Input: part model. Units: mm. Frame: model coordinates. A direction names the side the tool comes from. Coordinates: 2 decimals unless noted, no trailing zeros. One line per question, with ' | ' between items.
from build123d import *

# Parameters (mm, degrees)
F1_DEPTH  = 3.175
F2_W      = 25.4
F2_H      = 6.35
F3_DEPTH  = 12.7
F5_DEPTH  = 6.35
F7_DEPTH  = 6.35
F10_DEPTH = 6.35
F13_R     = 0.873125
F14_DEPTH = 25.4


with BuildPart() as f1:
    # F0 (on Front) → F1 (new body, symmetric)
    with BuildSketch(Plane.XZ):
        Polygon((3.175, 15.875), (0, 15.875), (-3.175, 15.875), (-12.7, 0), (12.7, 0), align=None)
        Polygon((12.7, -6.35), (12.7, 0), (-12.7, 0), (-12.7, -6.35), (0, -6.35), align=None)
        Polygon((0, -15.875), (12.7, -6.35), (0, -6.35), align=None)
        Polygon((0, -6.35), (-12.7, -6.35), (0, -15.875), align=None)
    extrude(amount=F1_DEPTH, both=True)

    # F2 (on face) → F3 (join)
    with BuildSketch(Plane.XZ.offset(3.175)):
        with Locations((0, -3.175)):
            Rectangle(F2_W, F2_H)
    extrude(amount=F3_DEPTH)

    # F4 (on face) → F5 (join)
    with BuildSketch(Plane(origin=(7.62, 0, -10.16), x_dir=(0.8, 0, 0.6), z_dir=(0.6, 0, -0.8))):
        Polygon((-9.525, 3.175), (6.35, 3.175), (6.35, 15.875), align=None)
    extrude(amount=-F5_DEPTH)

    # F6 (on face) → F7 (join)
    with BuildSketch(Plane(origin=(-7.62, 0, -10.16), x_dir=(0.8, 0, -0.6), z_dir=(-0.6, 0, -0.8))):
        Polygon((-6.35, 15.875), (-6.35, 3.175), (9.525, 3.175), align=None)
    extrude(amount=-F7_DEPTH)

    # F9 (on 3pt) → F10 (join)
    with BuildSketch(Plane(origin=(0, -8.763, -11.684), x_dir=(1, 0, 0), z_dir=(0, -0.6, -0.8))):
        Polygon((0, -6.9850953296), (12.700131163, 8.8898520917), (-12.699984014, 8.8898520917), align=None)
    extrude(amount=-F10_DEPTH)

    # F13 (on 3pt) → F14 (cut)
    with BuildSketch(Plane(origin=(0, -9.525, 9.525), x_dir=(1, 0, 0), z_dir=(0, -0.7071067812, 0.7071067812))):
        with Locations((0, 3.3772722036)):
            Circle(F13_R)
    extrude(amount=-F14_DEPTH, mode=Mode.SUBTRACT)


solid = f1.part
Item 1: Contact query for flat-ended pins moving along their axis: P1, Ø6, axis at y = -3.5, z = -12.5, coming from the +X side; P2, Ø12.5, axis at x = 0, z = 10.5, coming from the -Y side (3 decimals); P3, Ø1.1, axis at x = 0.5, y = -3.5, coming from the -Z side. Output: stop coordinate, or through.
Data:
P1: x = 8.5 | P2: y = -3.175 | P3: z = -15.85
Item 2: Access query for faces 1 (the face through (0, -3.175, 6)), 2 (the face through (0, -4, -6.35)), 3 (the face through (12.7, -6, -3)). Directions: +Z, -Z, +X, -X, +Y, -Y. A direction counts if a zero-diameter tool reaches every point of the face in a straight line with its end or side. Return the directions, or none.
Data:
face 1: +Z, +X, -X, -Y | face 2: none | face 3: +Z, -Z, +X, +Y, -Y
Item 3: Draft query along X for faces 4 (the face through (0, -9, 0)), 5 (the face through (8, -0.04, 7.83)), 6 (the face through (-7.9, 0, 8)), 7 (the face through (-0.03, -4.48, -6.96)). Return one class per face: released by +X, released by -X, zero draft, split by the parting line, or undercut.
Data:
face 4: zero draft | face 5: released by +X | face 6: released by -X | face 7: undercut
Item 4: Ray query, line 1 (Y direction, x = -2.75, z = 8) (3 decimals); line 2 (Z direction, x = -0.75, y = -5); line 3 (X direction, y = -0.5, z = -13.5). Return the intervals inside material, ascending.
Data:
line 1: -3.175 to 3.175 | line 2: -14.51 to -6.57, -6.35 to 0 | line 3: -3.17 to 3.17
